Design review of the part built by this model. Coordinates are the model's own, in mm. Face numbers are marked on the shaded views. A direction names the side the tool comes from. Round coordinates to 2 decimals unless told otherwise and drop trailing zeros. Loops run counter-clockwise (first coordinate to the right, second up) from the corner with the lowest first, then second, coordinate; pieces in that order, holes last. Notation, with made-up numbers: (27.25, -1.75) - (61.25, -1.75) arc R25 ccw to (61.25, 32.25) - close; hole circle Ø2 at (64, -14). An arc over 180 degrees is marked (long way). One line per question, with ' | ' between items. Start each with the question number.
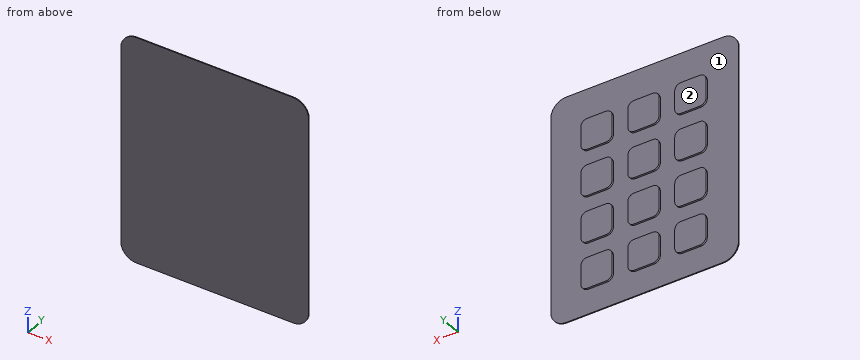
from build123d import *

# Parameters (mm, degrees)
SKETCH1_W              = 60
SKETCH1_H              = 73
BOSS_EXTRUDE1_DEPTH    = 0.3
FILLET1_R              = 5
SKETCH2_W              = 10
SKETCH2_H              = 10
BOSS_EXTRUDE2_DEPTH    = 0.6
FILLET2_R              = 2
LPATTERN1_COUNT        = 3
LPATTERN1_PITCH        = 15
LPATTERN1_COUNT_DIR2   = 4
LPATTERN1_PITCH_DIR2   = 15
FILLET2_OF_LPATTERN1_R = 2


with BuildPart() as part:
    # Sketch1 → Boss-Extrude1 (new body)
    with BuildSketch(Plane(origin=(0, 0, 0), x_dir=(1, 0, 0), z_dir=(0, 1, 0))):
        with Locations((-13.75, 5.339285714)):
            Rectangle(SKETCH1_W, SKETCH1_H)
    extrude(amount=BOSS_EXTRUDE1_DEPTH)

    # Fillet1
    fillet1_edges = [part.edges().sort_by_distance(p)[0] for p in [
        (-43.75, 0.15, -41.839285714),
        (16.25, 0.15, -41.839285714),
        (16.25, 0.15, 31.160714286),
        (-43.75, 0.15, 31.160714286),
    ]]
    fillet(fillet1_edges, radius=FILLET1_R)

    # Sketch2 → Boss-Extrude2 (add)
    with BuildSketch(Plane(origin=(0, 0.3, 0), x_dir=(1, 0, 0), z_dir=(0, 1, 0))):
        with Locations((1.25, -16.160714286)):
            Rectangle(SKETCH2_W, SKETCH2_H)
    boss_extrude2 = extrude(amount=BOSS_EXTRUDE2_DEPTH)

    # Fillet2
    fillet2_edges = [part.edges().sort_by_distance(p)[0] for p in [
        (6.25, 0.6, 21.160714286),
        (6.25, 0.6, 11.160714286),
        (-3.75, 0.6, 11.160714286),
        (-3.75, 0.6, 21.160714286),
    ]]
    fillet(fillet2_edges, radius=FILLET2_R)

    # LPattern1: Boss-Extrude2 3 × 4
    with Locations(*[(-i * LPATTERN1_PITCH, 0, -j * LPATTERN1_PITCH_DIR2) for i in range(LPATTERN1_COUNT) for j in range(LPATTERN1_COUNT_DIR2) if (i, j) != (0, 0)]):
        add(boss_extrude2)

    # Fillet2 of LPattern1
    fillet2_of_lpattern1_edges = [part.edges().sort_by_distance(p)[0] for p in [
        (6.25, 0.6, 6.160714286),
        (6.25, 0.6, -3.839285714),
        (-3.75, 0.6, -3.839285714),
        (-3.75, 0.6, 6.160714286),
        (6.25, 0.6, -8.839285714),
        (6.25, 0.6, -18.839285714),
        (-3.75, 0.6, -18.839285714),
        (-3.75, 0.6, -8.839285714),
        (6.25, 0.6, -23.839285714),
        (6.25, 0.6, -33.839285714),
        (-3.75, 0.6, -33.839285714),
        (-3.75, 0.6, -23.839285714),
        (-8.75, 0.6, 21.160714286),
        (-8.75, 0.6, 11.160714286),
        (-18.75, 0.6, 11.160714286),
        (-18.75, 0.6, 21.160714286),
        (-8.75, 0.6, 6.160714286),
        (-8.75, 0.6, -3.839285714),
        (-18.75, 0.6, -3.839285714),
        (-18.75, 0.6, 6.160714286),
        (-8.75, 0.6, -8.839285714),
        (-8.75, 0.6, -18.839285714),
        (-18.75, 0.6, -18.839285714),
        (-18.75, 0.6, -8.839285714),
        (-8.75, 0.6, -23.839285714),
        (-8.75, 0.6, -33.839285714),
        (-18.75, 0.6, -33.839285714),
        (-18.75, 0.6, -23.839285714),
        (-23.75, 0.6, 21.160714286),
        (-23.75, 0.6, 11.160714286),
        (-33.75, 0.6, 11.160714286),
        (-33.75, 0.6, 21.160714286),
        (-23.75, 0.6, 6.160714286),
        (-23.75, 0.6, -3.839285714),
        (-33.75, 0.6, -3.839285714),
        (-33.75, 0.6, 6.160714286),
        (-23.75, 0.6, -8.839285714),
        (-23.75, 0.6, -18.839285714),
        (-33.75, 0.6, -18.839285714),
        (-33.75, 0.6, -8.839285714),
        (-23.75, 0.6, -23.839285714),
        (-23.75, 0.6, -33.839285714),
        (-33.75, 0.6, -33.839285714),
        (-33.75, 0.6, -23.839285714),
    ]]
    fillet(fillet2_of_lpattern1_edges, radius=FILLET2_OF_LPATTERN1_R)


solid = part.part
1. To check wall thickness, follow line 1 along Z through (x, y) = (-15, 0.5); line 2 along X through (y, z) = (0.45, -30.5); line 3 along X through (y, z) = (0.4, -17). State the ranges of each line that lie inside material, in increasing order.
2. Take a section at B-B, the plane y = 0.5. Count the separate pieces of the cut face and the enclosed holes in it, then the cut area to 3 significant figures.
3. Machinability: for the marked faces 1 and 2, which of the approach directions +Z, -Z, +X, -X, +Y, -Y give a long, thin tool a straight path to every point of the face, cutting with its end or side? Answer none if there is none.
4. Take a section at A-A, the plane z = -29.5. Give the boundary of the cut face in (x, y), then the cut area to 3 significant figures.
5. Take a section at D-D, the plane x = -20.5. Give the boundary of the cut face in (y, z), then the cut area to 3 significant figures.
6. Clearance check with a flat-ended pin moving along its axis: P1, Ø3, axis at x = -8, z = 10.5, coming from the +Y side. State where the tip first meets the part, or that it passes through.
7. Take a section at C-C, the plane x = -29. Give the boundary of the cut face in (y, z).
Answer list:
1) line 1: z = -33.84 to -23.84, -18.84 to -8.84, -3.84 to 6.16, 11.16 to 21.16 | line 2: x = -33.75 to -23.75, -18.75 to -8.75, -3.75 to 6.25 | line 3: x = -33.74 to -23.76, -18.74 to -8.76, -3.74 to 6.24
2) separate pieces: 12 | enclosed holes: 0 | area: 1,160 mm²
3) face 1: +Y | face 2: +Z, -Z, +X, -X, +Y
4) outline: (-43.75, 0) - (16.25, 0) - (16.25, 0.3) - (6.25, 0.3) - (6.25, 0.9) - (-3.75, 0.9) - (-3.75, 0.3) - (-8.75, 0.3) - (-8.75, 0.9) - (-18.75, 0.9) - (-18.75, 0.3) - (-23.75, 0.3) - (-23.75, 0.9) - (-33.75, 0.9) - (-33.75, 0.3) - (-43.75, 0.3) - close | area: 36.0 mm²
5) outline: (0, -41.84) - (0.3, -41.84) - (0.3, 31.16) - (0, 31.16) - close | area: 21.9 mm²
6) P1: stops at y = 0.3
7) outline: (0, -41.84) - (0.3, -41.84) - (0.3, -33.84) - (0.9, -33.84) - (0.9, -23.84) - (0.3, -23.84) - (0.3, -18.84) - (0.9, -18.84) - (0.9, -8.84) - (0.3, -8.84) - (0.3, -3.84) - (0.9, -3.84) - (0.9, 6.16) - (0.3, 6.16) - (0.3, 11.16) - (0.9, 11.16) - (0.9, 21.16) - (0.3, 21.16) - (0.3, 31.16) - (0, 31.16) - close
